Check sheet for the modelled part. Datum: model origin and axes. Units: mm. Face numbers are marked on the shaded views. A direction names the side the tool comes from. Round coordinates to 2 decimals unless told otherwise and drop trailing zeros. Write each loop counter-clockwise with the first axis right and the second up, starting at its lowest first coordinate (ties: lowest second). Pieces come first, ordered by that corner, then holes. Notation, with made-up numbers: M 59.5,-10 L 88.5,-10 A25 cw 88.5,29 Z; hole C -18,31 d3. An arc over 180 degrees is marked long. Put each result on its own line as item: value.
```python
from build123d import *

# Parameters (mm, degrees)
F1_DEPTH = 14.5
F4_DEPTH = 5.5
F5_R     = 1.4
F6_DEPTH = 9.5
F7_R     = 4
F8_DEPTH = 1
F9_R     = 1


with BuildPart() as f1:
    # F0 (on Front) → F1 (new body)
    with BuildSketch(Plane.XZ):
        with BuildLine():
            ThreePointArc((0, 3.15), (2.2273863607, 2.2273863607), (3.15, 0))
            ThreePointArc((3.15, 0), (2.2273863607, -2.2273863607), (0, -3.15))
            Line((0, -3.15), (0, -5.15))
            Line((0, -5.15), (10, -5.15))
            Line((10, -5.15), (10, 0))
            Line((10, 0), (10, 5.15))
            Line((10, 5.15), (0, 5.15))
            Line((0, 5.15), (0, 3.15))
        make_face()
        with BuildLine():
            ThreePointArc((0, -3.15), (-3.15, 0), (0, 3.15))
            Line((0, 3.15), (0, 5.15))
            ThreePointArc((0, 5.15), (-5.15, 0), (0, -5.15))
            Line((0, -5.15), (0, -3.15))
        make_face()
    extrude(amount=F1_DEPTH)

    # F3 (on offset) → F4 (cut)
    with BuildSketch(Plane.XZ.offset(12.5)):
        Polygon((-9.8062800243, -5.15), (0, -5.15), (3.4, -5.15), (10, 1.45), (10, 5.7288180105), (-9.8062800243, 5.7288180105), align=None)
    extrude(amount=-F4_DEPTH, mode=Mode.SUBTRACT)

    # F5 (on face) → F6 (cut)
    with BuildSketch(Plane.YZ.offset(10)):
        with Locations((-3.5, 0)):
            Circle(F5_R)
    extrude(amount=-F6_DEPTH, mode=Mode.SUBTRACT)

    # F7 (on face) → F8 (join)
    with BuildSketch(Plane(origin=(0, 0, 0), x_dir=(-1, 0, 0), z_dir=(0, 1, 0))):
        Circle(F7_R)
    extrude(amount=-F8_DEPTH)

    # F9
    f9_edges = [f1.edges().sort_by_distance(p)[0] for p in [
        (10, -13.5, 5.15),
        (10, -3.5, 5.15),
    ]]
    fillet(f9_edges, radius=F9_R)


solid = f1.part
```
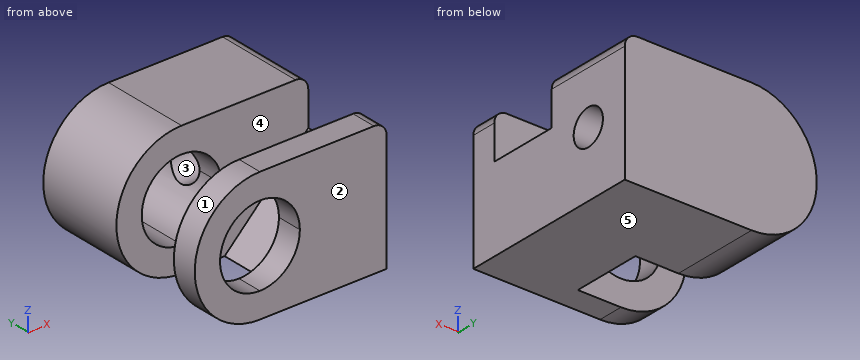
1. Depth check by flat-ended pin: pin 1 Ø5 at (y, z) = (-12.5, -3) entering from -X; pin 2 Ø4 at (x, y) = (-3, -11) entering from -Z. Enter the tip coordinate at first touch or a pass-through.
Computed values:
pin 1: stops at x = -5.13
pin 2: stops at z = -4.87
2. Release check for a two-part mould opening along Y. For the marked faces 1, 2 and 3 record: +Y half, -Y half, draft (parallel to the pull), parting line (faces both ways), or undercut.
Computed values:
face 1: draft
face 2: -Y half
face 3: undercut
3. Cross-section at C-C (y = -3.5). Enter the section's corners in (x, z), then the cut area to 3 significant figures.
Computed values:
outline: M 0,-5.15 L 10,-5.15 L 10,-1.4 L 2.82,-1.4 A3.15 cw long 2.82,1.4 L 10,1.4 L 10,4.15 A1 ccw 9,5.15 L 0,5.15 A5.15 ccw Z
area: 93.8 mm2
4. Cross-section at A-A (y = -1.5). Enter the section's corners in (x, z).
Computed values:
outline: M 0,-5.15 L 10,-5.15 L 10,4.15 A1 ccw 9,5.15 L 0,5.15 A5.15 ccw Z; hole C 0,0 d6.3
5. Cross-section at B-B (x = 7). Enter the section's corners in (y, z), then the cut area to 3 significant figures.
Computed values:
outline: M -14.5,-5.15 L 0,-5.15 L 0,5.15 L -7,5.15 L -7,-1.55 L -12.5,-1.55 L -12.5,5.15 L -14.5,5.15 Z; hole C -3.5,0 d2.8
area: 106 mm2
6. Cross-section at D-D (x = 1.5). Enter the section's corners in (y, z).
Computed values:
outline: M -14.5,-5.15 L -12.5,-5.15 L -12.5,-2.77 L -14.5,-2.77 Z; M -14.5,2.77 L -12.5,2.77 L -12.5,5.15 L -14.5,5.15 Z; M -7,-5.15 L 0,-5.15 L 0,5.15 L -7,5.15 L -7,2.77 L -1,2.77 L -1,-2.77 L -7,-2.77 Z
7. Access from +Z, -Z, +X, -X, +Y, -Y to the whole of each face (thin tool, end or side, straight path). Record for the marked faces 4 and 5.
Computed values:
face 4: +Z, -X
face 5: -Z, +X, -X, +Y, -Y
8. Scan lines: probe 1 along Z at (x, y) = (4.5, -3.5); probe 2 along Y at (x, z) = (2.75, 4); probe 3 along Y at (x, z) = (8.5, -0.25). Record each from-to range of solid material in increasing order.
Computed values:
probe 1: z = -5.15 to -1.4, 1.4 to 5.15
probe 2: y = -14.5 to -12.5, -7 to 0
probe 3: y = -14.5 to -4.88, -2.12 to 0
